```python
from build123d import *

# Parameters (mm, degrees)
SKETCH1_R           = 11
SKETCH1_R_2         = 3.5
BOSS_EXTRUDE1_DEPTH = 3.75
CHAMFER1_SIZE       = 0.75
SKETCH2_R           = 9
CUT_EXTRUDE1_DEPTH  = 1.75
CHAMFER2_SIZE       = 0.75


with BuildPart() as part:
    # Sketch1 → Boss-Extrude1 (new body)
    with BuildSketch(Plane.XY):
        Circle(SKETCH1_R)
        Circle(SKETCH1_R_2, mode=Mode.SUBTRACT)
    extrude(amount=BOSS_EXTRUDE1_DEPTH)

    # Chamfer1
    chamfer1_edges = [part.edges().sort_by_distance(p)[0] for p in [
        (-11, 0, 0),
    ]]
    chamfer(chamfer1_edges, length=CHAMFER1_SIZE)

    # Sketch2 → Cut-Extrude1 (cut)
    with BuildSketch(Plane.XY.offset(3.75)):
        Circle(SKETCH2_R)
    extrude(amount=-CUT_EXTRUDE1_DEPTH, mode=Mode.SUBTRACT)

    # Chamfer2
    chamfer2_edges = [part.edges().sort_by_distance(p)[0] for p in [
        (-9, 0, 2),
    ]]
    chamfer(chamfer2_edges, length=CHAMFER2_SIZE)


solid = part.part
```
The model under review builds one solid part; all positions refer to its coordinate system, in mm. A direction names the side the tool comes from. Give positions to 0.01 mm unless a question says otherwise; leave off trailing zeros. Write each loop counter-clockwise with the first axis right and the second up, starting at its lowest first coordinate (ties: lowest second). Pieces come first, ordered by that corner, then holes. Notation, with made-up numbers: M 67.25,-18.75 L 71.25,-18.75 A17 ccw 71.25,10.25 Z; hole C -10.5,-26.5 d3. An arc over 180 degrees is marked long. Write each question's results on one line, items separated by ' | '. Start each with the question number.
1. Insertion check: pin 1 Ø2 at (x, z) = (6.5, 2.5) entering from +Y; pin 2 Ø8 at (x, y) = (4, 1) entering from +Z; pin 3 Ø2 at (y, z) = (-0.5, 0.5) entering from +X; pin 4 Ø1 at (x, y) = (1, -0.5) entering from -Z. Each pin has a flat end and moves straight along its axis. Give the tip position at first contact, or say it passes through.
2. We need section C-C (z = 1.3). Write out the cut boundary in (x, y), and give its area (3 significant figures).
3. For faces 1 (the flat face through (2, -9, 3.75)), 2 (the cylindrical face through (-1.172, 8.923, 3.257)), list the 3-axis set-ups (+Z, -Z, +X, -X, +Y, -Y) from which the entire face can be reached by the end or side of a thin tool; tool diameter is ignored.
4. We need section A-A (x = 0). Write out the cut boundary in (y, z), and give its area (3 significant figures).
5. For probe 1 along Y at (x, z) = (0, 3.25); probe 2 along Y at (x, z) = (0, 1.25); probe 3 along Z at (x, y) = (2.25, -7.25), list the stretches that pass through material, from the lowest coordinate up. Write a range as [from, to].
Results found:
1) pin 1: stops at y = 9.53 | pin 2: stops at z = 2 | pin 3: stops at x = 11 | pin 4: passes through
2) outline: C 0,0 d22; hole C 0,0 d7 | area: 342 mm^2
3) face 1: +Z, +X, -X, +Y, -Y | face 2: +Z
4) outline: M -11,0.75 L -10.25,0 L -3.5,0 L -3.5,2 L -8.25,2 L -9,2.75 L -9,3.75 L -11,3.75 Z; M 3.5,0 L 10.25,0 L 11,0.75 L 11,3.75 L 9,3.75 L 9,2.75 L 8.25,2 L 3.5,2 Z | area: 37.0 mm^2
5) probe 1: y = [-11, -9], [9, 11] | probe 2: y = [-11, -3.5], [3.5, 11] | probe 3: z = [0, 2]
